Solid Edge part; units mm, degrees
sketch "Sketch1" plane through (0, 0, 0) normal (0, -1, 0) x (1, 0, 0)
  circle A0 centre (0, 0) radius 50
  circle A1 centre (0, 0) radius 40
extrude "Protrusion1" add sketch "Sketch1" along normal mid plane 6
sketch "Sketch2" plane through (0, -3, 0) normal (0, -1, 0) x (1, 0, 0)
  line L0 (32, 8) -> (47, 8)
  line L1 (47, 8) -> (47, -8)
  line L2 (47, -8) -> (32, -8)
  line L3 (32, -8) -> (32, 8)
extrude "Protrusion2" add sketch "Sketch2" against normal up to vertex (6 mm away)
pattern_circular "Pattern1" count 3 over 360 about axis through (0, -3, 0) along (0, -1, 0) of "Protrusion2"
sketch "Sketch3" plane through (0, -3, 0) normal (0, -1, 0) x (1, 0, 0)
  line L0 (42, 3) -> (42, -3)
  line L1 (42, -3) -> (37, -3)
  line L2 (37, -3) -> (37, 3)
  line L3 (37, 3) -> (42, 3)
extrude "Cutout1" cut sketch "Sketch3" against normal up to vertex (6 mm away)
pattern_circular "Pattern2" count 3 over 360 about axis through (0, -3, 0) along (0, -1, 0) of "Cutout1"
Model file for the job. Use its own axes, mm. A direction names the side the tool comes from. Give positions to 0.01 mm unless a question says otherwise; leave off trailing zeros. Order: outer loops, then holes, each group sorted by start corner. A loop starts at its lowest first (then second) coordinate and runs counter-clockwise, first axis right, second up. Notation, with made-up numbers: M -24,88 L -15,88 A30 cw -15,110 Z; hole C -19.75,-31 d8. An arc over 180 degrees is marked long. Write item = value, one per line.
Q1. Drill centre lines: line 1 (Z direction, x = 0.5, y = 1.2); line 2 (X direction, y = -2.7, z = -32.5); line 3 (Z direction, x = -23, y = -2.35). Where is each one in solid material? Low to high. Write a range as [from, to].
Derived:
line_1 = [-50, -40], [40, 50]
line_2 = [-38, -22.23], [-17.71, -9.53], [23.32, 38]
line_3 = [-44.4, -35.22], [-33.84, -23.84], [23.84, 33.84], [35.22, 44.4]
Q2. Flat gauge pins, fed straight in: pin 1 (3 mm diameter, centred on y = 0.5, z = -2.5, fed in from -X); pin 2 (2 mm diameter, centred on x = -26, y = -0.5, fed in from -Z); pin 3 (2 mm diameter, centred on x = 12.5, y = 2, fed in from +Z). Where does each tip first touch, or does it go through?
Derived:
pin_1 = -49.99
pin_2 = -43.3
pin_3 = 48.66
Q3. Cut at C-C, the plane y = -1.2. List the corners of the cut face in (x, z), then the cut area to 3 significant figures.
Derived:
outline = C 0,0 d100; hole M -26.52,-29.94 L -22.93,-23.71 L -9.07,-31.71 L -12.67,-37.94 A40 ccw 39.19,-8 L 32,-8 L 32,8 L 39.19,8 A40 ccw -12.67,37.94 L -9.07,31.71 L -22.93,23.71 L -26.52,29.94 A40 ccw Z; hole M -23.6,-34.87 L -18.4,-37.87 L -15.9,-33.54 L -21.1,-30.54 Z; hole M -23.6,34.87 L -21.1,30.54 L -15.9,33.54 L -18.4,37.87 Z; hole M 37,-3 L 42,-3 L 42,3 L 37,3 Z
area = 3,110 mm2
Q4. Cut at D-D, the plane z = -16. List the corners of the cut face in (x, y).
Derived:
outline = M -47.37,-3 L -36.66,-3 L -36.66,3 L -47.37,3 Z; M 36.66,-3 L 47.37,-3 L 47.37,3 L 36.66,3 Z
Q5. Two-plate mould, pull along Z, no slides. Class faces 3 (the cylindrical face through (47.69, -0.04, 15.02)), 4 (the flat face through (34, -3, -3)), 5 (the flat face through (39, 0, 3)): pulls with the +Z half, pulls with the -Z half, needs draft (parallel to the pull), parting line crosses it, or undercut.
Derived:
face_3 = parting line crosses it
face_4 = needs draft
face_5 = undercut
Q6. Tool access for faces 1 (the flat face through (-18.464, -0.042, 32.064)), 2 (the flat face through (-14, 3, -31)): list every direction of +Z, -Z, +X, -X, +Y, -Y with a clear straight run to the whole face (end or side of a thin tool).
Derived:
face_1 = +Y, -Y
face_2 = +Z, -Z, +X, -X, +Y
Q7. Cut at A-A, the plane x = 0. List the corners of the cut face in (y, z), then the cut area to 3 significant figures.
Derived:
outline = M -3,-50 L 3,-50 L 3,-40 L -3,-40 Z; M -3,40 L 3,40 L 3,50 L -3,50 Z
area = 120 mm2
Q8. Cut at B-B, the plane z = 0. List the corners of the cut face in (x, y), then the cut area to 3 significant figures.
Derived:
outline = M -50,-3 L -40,-3 L -40,3 L -50,3 Z; M 32,-3 L 37,-3 L 37,3 L 32,3 Z; M 42,-3 L 50,-3 L 50,3 L 42,3 Z
area = 138 mm2
